from build123d import *

# Parameters (mm, degrees)
SKETCH4_R             = 9
BOSS_EXTRUDE1_DEPTH   = 15
SKETCH5_R             = 4
CUT_EXTRUDE1_DEPTH    = 7
SKETCH6_R             = 2.25
CUT_EXTRUDE2_DEPTH    = 9
BOSS_EXTRUDE3_DEPTH   = 5
CHAMFER1_SIZE         = 2
M4_TAPPED_HOLE1_D     = 3.3
M4_TAPPED_HOLE1_DEPTH = 8
M4_TAPPED_HOLE1_TIP   = 0.991420021


with BuildPart() as part:
    # Sketch4 → Boss-Extrude1 (new body)
    with BuildSketch(Plane.XY):
        Polygon((-38.333333333, -25.277777778), (-38.333333333, 24.722222222), (-18.333333333, 24.722222222), (-18.333333333, 19.722222222), (-5.333333333, 19.722222222), (-5.333333333, 9.722222222), (-5.833333333, 9.722222222), (-5.833333333, -10.277777778), (-5.333333333, -10.277777778), (-5.333333333, -20.277777778), (-18.333333333, -20.277777778), (-18.333333333, -25.277777778), align=None)
        with Locations((-23.608519649, -0.277777778)):
            Circle(SKETCH4_R, mode=Mode.SUBTRACT)
    extrude(amount=BOSS_EXTRUDE1_DEPTH)

    # Sketch5 → Cut-Extrude1 (cut)
    with BuildSketch(Plane(origin=(0, 0, 0), x_dir=(-1, 0, 0), z_dir=(0, 0, -1))):
        with Locations((30.333333333, 17.722222222)):
            Circle(SKETCH5_R)
        with Locations((30.333333333, -18.277777778)):
            Circle(SKETCH5_R)
    extrude(amount=-CUT_EXTRUDE1_DEPTH, mode=Mode.SUBTRACT)

    # Sketch6 → Cut-Extrude2 (cut, through all)
    with BuildSketch(Plane(origin=(0, 0, 7), x_dir=(-1, 0, 0), z_dir=(0, 0, -1))):
        with Locations((30.333333333, 17.722222222)):
            Circle(SKETCH6_R)
        with Locations((30.333333333, -18.277777778)):
            Circle(SKETCH6_R)
    extrude(amount=-CUT_EXTRUDE2_DEPTH, mode=Mode.SUBTRACT)

    # Sketch9 → Boss-Extrude3 (add)
    with BuildSketch(Plane(origin=(0, 0, 0), x_dir=(-1, 0, 0), z_dir=(0, 0, -1))):
        Polygon((13.333333333, -20.277777778), (5.333333333, -20.277777778), (5.333333333, -10.277777778), (5.833333333, -10.277777778), (5.833333333, 9.722222222), (5.333333333, 9.722222222), (5.333333333, 19.722222222), (13.333333333, 19.722222222), align=None)
    extrude(amount=BOSS_EXTRUDE3_DEPTH)

    # Chamfer1
    chamfer1_edges = [part.edges().sort_by_distance(p)[0] for p in [
        (-38.333333333, -25.277777778, 7.5),
        (-38.333333333, 24.722222222, 7.5),
    ]]
    chamfer(chamfer1_edges, length=CHAMFER1_SIZE)

    # M4 Tapped Hole1
    with Locations(Plane(origin=(-5.333333333, 0, 0), x_dir=(0, 0, -1), z_dir=(1, 0, 0))):
        with Locations((-5, 14.722222222), (-5, -15.277777778)):
            Hole(M4_TAPPED_HOLE1_D / 2, depth=M4_TAPPED_HOLE1_DEPTH)
            with Locations((0, 0, -(M4_TAPPED_HOLE1_DEPTH + M4_TAPPED_HOLE1_TIP / 2))):  # 118° drill point
                Cone(0, M4_TAPPED_HOLE1_D / 2, M4_TAPPED_HOLE1_TIP, mode=Mode.SUBTRACT)


solid = part.part
Input: part model. Units: mm. Frame: model coordinates. A direction names the side the tool comes from. Give positions to 0.01 mm unless a question says otherwise; leave off trailing zeros. Order: outer loops, then holes, each group sorted by start corner. A loop starts at its lowest first (then second) coordinate and runs counter-clockwise, first axis right, second up. Notation, with made-up numbers: (10.25, 41) - (48.25, 41) arc R20 ccw to (48.25, 61) - close; hole circle Ø3 at (84, -35.5). An arc over 180 degrees is marked (long way). Write each question's results on one line, items separated by ' | '.
Item 1: Section C-C (z = 2). Return loops of the section in (x, y), and give its area (3 significant figures).
A:
outline: (-38.33, -23.28) - (-36.33, -25.28) - (-18.33, -25.28) - (-18.33, -20.28) - (-5.33, -20.28) - (-5.33, -10.28) - (-5.83, -10.28) - (-5.83, 9.72) - (-5.33, 9.72) - (-5.33, 19.72) - (-18.33, 19.72) - (-18.33, 24.72) - (-36.33, 24.72) - (-38.33, 22.72) - close; hole circle Ø8 at (-30.33, -18.28); hole circle Ø8 at (-30.33, 17.72); hole circle Ø18 at (-23.61, -0.28) | area: 1,150 mm^2
Item 2: Material intervals for line 1 along Y through (x, z) = (-10, 5); line 2 along Y through (x, z) = (-31.5, 13.5); line 3 along X through (y, z) = (3.5, -2.5), sorted ascending.
A:
line 1: y = -20.28 to -16.93, -13.63 to 13.07, 16.37 to 19.72 | line 2: y = -25.28 to -20.2, -16.35 to -4.6, 4.05 to 15.8, 19.65 to 24.72 | line 3: x = -13.33 to -5.83
Item 3: Draft query along Z for faces 5 (the flat face through (-27, -25.278, 7)), 6 (the cylindrical face through (-9.39, -16.89, 4.64)), 7 (the flat face through (-14, 0, 15)). Return one class per face: released by +Z, released by -Z, zero draft, split by the parting line, or undercut.
A:
face 5: zero draft | face 6: undercut | face 7: released by +Z
Item 4: Section A-A (y = 3). Return loops of the section in (x, z).
A:
outline: (-38.33, 0) - (-31.99, 0) - (-31.99, 15) - (-38.33, 15) - close; (-15.23, 0) - (-13.33, 0) - (-13.33, -5) - (-5.83, -5) - (-5.83, 15) - (-15.23, 15) - close
Item 5: Access query for faces 1 (the flat face through (-5.833, 0, 5)), 2 (the flat face through (-31, 6, 0)), 3 (the flat face through (-32.1, 16, 7)), 4 (the flat face through (-18.333, -23, 7)). Directions: +Z, -Z, +X, -X, +Y, -Y. A direction counts if a zero-diameter tool reaches every point of the face in a straight line with its end or side. Return the directions, or none.
A:
face 1: +Z, -Z, +X | face 2: -Z, -X, +Y, -Y | face 3: -Z | face 4: +Z, -Z, +X, -Y
Item 6: Section B-B (x = -24). Return loops of the section in (y, z).
A:
outline: (-25.28, 0) - (-9.27, 0) - (-9.27, 15) - (-25.28, 15) - close; (8.71, 0) - (24.72, 0) - (24.72, 15) - (8.71, 15) - close
Item 7: Contact query for flat-ended pins moving along their axis: pin 1 Ø9 at (x, y) = (-28.5, -19.5) entering from -Z; pin 2 Ø6 at (y, z) = (-4, -0.5) entering from +X; pin 3 Ø2.5 at (y, z) = (-23.5, 9) entering from +X; pin 4 Ø5 at (x, y) = (-30.33, -18.28) entering from +Z. Output: stop coordinate, or through.
A:
pin 1: stops at z = 0 | pin 2: stops at x = -5.83 | pin 3: stops at x = -18.33 | pin 4: stops at z = 15
Item 8: Section D-D (x = -17). Return loops of the section in (y, z), and give its area (3 significant figures).
A:
outline: (-20.28, 0) - (-6.39, 0) - (-6.39, 15) - (-20.28, 15) - close; (5.83, 0) - (19.72, 0) - (19.72, 15) - (5.83, 15) - close | area: 417 mm^2
